Check sheet for the modelled part. Datum: model origin and axes. Units: mm. A direction names the side the tool comes from. Give positions to 0.01 mm unless a question says otherwise; leave off trailing zeros. Write each loop counter-clockwise with the first axis right and the second up, starting at its lowest first coordinate (ties: lowest second). Pieces come first, ordered by that corner, then holes. Notation, with made-up numbers: M 61,1 L 87,1 A31 cw 87,35 Z; hole C 28,17 d9. An arc over 180 degrees is marked long. One line per item, written item: value. Start each with the question number.
from build123d import *

# Parameters (mm, degrees)
SKETCH1_R           = 10.9
BOSS_EXTRUDE1_DEPTH = 245
SKETCH2_R           = 10.9
SKETCH2_R_2         = 6
CUT_EXTRUDE1_DEPTH  = 20
CUT_EXTRUDE2_START  = -20
SKETCH4_R           = 10.9
SKETCH4_R_2         = 6
CUT_EXTRUDE2_DEPTH  = 20
CHAMFER1_SIZE       = 2


with BuildPart() as part:
    # Sketch1 → Boss-Extrude1 (new, symmetric)
    with BuildSketch(Plane(origin=(0, 0, 0), x_dir=(0, 0, -1), z_dir=(1, 0, 0))):
        Circle(SKETCH1_R)
    extrude(amount=BOSS_EXTRUDE1_DEPTH, both=True)

    # Sketch2 → Cut-Extrude1 (cut)
    with BuildSketch(Plane(origin=(245, 0, 0), x_dir=(0, 0, -1), z_dir=(1, 0, 0))):
        Circle(SKETCH2_R)
        Circle(SKETCH2_R_2, mode=Mode.SUBTRACT)
    extrude(amount=-CUT_EXTRUDE1_DEPTH, mode=Mode.SUBTRACT)

    # Sketch4 → Cut-Extrude2 (cut)
    with BuildSketch(Plane.ZY.offset(245).offset(CUT_EXTRUDE2_START)):
        Circle(SKETCH4_R)
        with Locations(Location((0, 0, 0), (0, 0, 180))):
            Circle(SKETCH4_R_2, mode=Mode.SUBTRACT)
    extrude(amount=CUT_EXTRUDE2_DEPTH, mode=Mode.SUBTRACT)

    # Chamfer1
    chamfer1_edges = [part.edges().sort_by_distance(p)[0] for p in [
        (-225, 0, 10.9),
        (225, 0, 10.9),
    ]]
    chamfer(chamfer1_edges, length=CHAMFER1_SIZE)


solid = part.part
1) Tool access check on faces 1 (the cylindrical face through (3.12, 3.27, -10.4)), 2 (the flat face through (225, -6, -2)), 3 (the cylindrical face through (-234.86, -1.802, -5.723)). Record the directions out of +Z, -Z, +X, -X, +Y, -Y that give a thin tool (end or side, any length) a straight path to the whole face; none if there is none.
2) Gauge pin test, flat ends, axial feed: pin 1 (3 mm diameter, centred on x = 72, z = 3.5, fed in from -Y); pin 2 (1.5 mm diameter, centred on y = 7.5, z = 1.5, fed in from -X); pin 3 (1.5 mm diameter, centred on x = 53.5, y = -5.5, fed in from +Z). Record the tip position at first contact, or that the pin passes through.
3) Cross-section at A-A (z = 0). Record the boundary of the cut face in (x, y).
4) Cross-section at C-C (x = -133.5). Record the boundary of the cut face in (y, z).
5) Material ranges on L1, parallel to Y at x = -112.5, z = 1; L2, parallel to Y at x = 141.5, z = -6.25; L3, parallel to X at y = -5.75, z = 5, recorded low to high. Write a range as from..to.
Data:
1. face 1: +X, -X
1. face 2: +X
1. face 3: -X
2. pin 1: stops at y = -10.71
2. pin 2: stops at x = -225
2. pin 3: stops at z = 9.81
3. outline: M -245,-6 L -225,-6 L -225,-8.9 L -223,-10.9 L 223,-10.9 L 225,-8.9 L 225,-6 L 245,-6 L 245,6 L 225,6 L 225,8.9 L 223,10.9 L -223,10.9 L -225,8.9 L -225,6 L -245,6 Z
4. outline: C 0,0 d21.8
5. L1: y = -10.85..10.85
5. L2: y = -8.93..8.93
5. L3: x = -225..225
